from build123d import *

# Parameters (mm, degrees)
F0_R     = 41.275
F1_DEPTH = 1.524
F2_R     = 2.2479
F3_DEPTH = 1.524
F4_R     = 29.3751
F5_DEPTH = 1.524


with BuildPart() as f1:
    # F0 (on Top) → F1 (new body)
    with BuildSketch(Plane.XY):
        Circle(F0_R)
    extrude(amount=F1_DEPTH)

    # F2 (on face) → F3 (cut, through all)
    with BuildSketch(Plane.XY.offset(1.524)):
        with Locations((0, 36.5252)):
            Circle(F2_R)
        with Locations((-31.631751, 18.2626)):
            Circle(F2_R)
        with Locations((-31.631751, -18.2626)):
            Circle(F2_R)
        with Locations((0, -36.5252)):
            Circle(F2_R)
        with Locations((31.631751, -18.2626)):
            Circle(F2_R)
        with Locations((31.631751, 18.2626)):
            Circle(F2_R)
    extrude(amount=-F3_DEPTH, mode=Mode.SUBTRACT)

    # F4 (on face) → F5 (cut, through all)
    with BuildSketch(Plane.XY.offset(1.524)):
        Circle(F4_R)
    extrude(amount=-F5_DEPTH, mode=Mode.SUBTRACT)


solid = f1.part
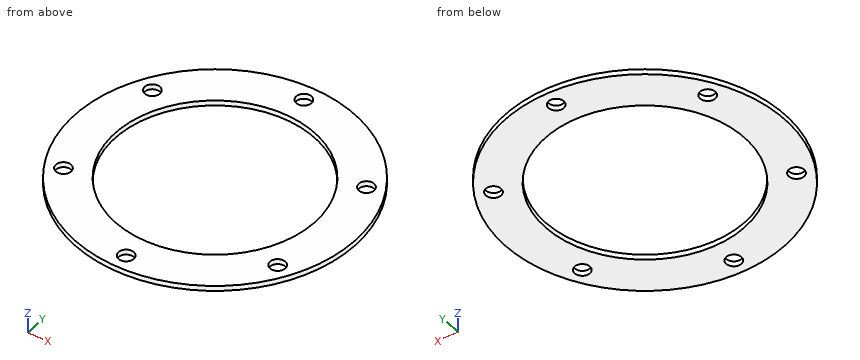
For this review, take the finished solid that the model builds, in its own axes (mm). Coordinates: 2 decimals unless noted, no trailing zeros. Loops run counter-clockwise (first coordinate to the right, second up) from the corner with the lowest first, then second, coordinate; pieces in that order, holes last. Notation, with made-up numbers: (1.5, 45.25) - (25.5, 45.25) arc R20 cw to (25.5, 55.25) - close; hole circle Ø7 at (84, 30). An arc over 180 degrees is marked (long way). Return JSON: item names as keys, results as strings.
Item 1: Take a section at C-C (z = 0.85). Give the boundary of the cut face in (x, y) (3 decimals), then the cut area to 3 significant figures.
Determined:
{"outline": "circle Ø82.55 at (0, 0); hole circle Ø4.496 at (-31.632, -18.263); hole circle Ø4.496 at (-31.632, 18.263); hole circle Ø58.75 at (0, 0); hole circle Ø4.496 at (0, -36.525); hole circle Ø4.496 at (0, 36.525); hole circle Ø4.496 at (31.632, -18.263); hole circle Ø4.496 at (31.632, 18.263)", "area": "2,550 mm2"}
Item 2: Take a section at A-A (y = 0). Give the boundary of the cut face in (x, z) (3 decimals), then the cut area to 3 significant figures.
Determined:
{"outline": "(-41.275, 0) - (-29.375, 0) - (-29.375, 1.524) - (-41.275, 1.524) - close; (29.375, 0) - (41.275, 0) - (41.275, 1.524) - (29.375, 1.524) - close", "area": "36.3 mm2"}
Item 3: Take a section at D-D (x = 32). Give the boundary of the cut face in (y, z).
Determined:
{"outline": "(-26.07, 0) - (-20.48, 0) - (-20.48, 1.52) - (-26.07, 1.52) - close; (-16.05, 0) - (16.05, 0) - (16.05, 1.52) - (-16.05, 1.52) - close; (20.48, 0) - (26.07, 0) - (26.07, 1.52) - (20.48, 1.52) - close"}
Item 4: Take a section at B-B (x = 0). Give the boundary of the cut face in (y, z) (3 decimals), then the cut area to 3 significant figures.
Determined:
{"outline": "(-41.275, 0) - (-38.773, 0) - (-38.773, 1.524) - (-41.275, 1.524) - close; (-34.277, 0) - (-29.375, 0) - (-29.375, 1.524) - (-34.277, 1.524) - close; (29.375, 0) - (34.277, 0) - (34.277, 1.524) - (29.375, 1.524) - close; (38.773, 0) - (41.275, 0) - (41.275, 1.524) - (38.773, 1.524) - close", "area": "22.6 mm2"}
Item 5: For line 1 (Y direction, x = 0, z = 1.05) (3 decimals); line 2 (X direction, y = -1, z = 0.9); line 3 (X direction, y = -16.5, z = 0.4), list the stretches that pass through material, from the lowest coordinate up.
Determined:
{"line 1": "y = -41.275 to -38.773, -34.277 to -29.375, 29.375 to 34.277, 38.773 to 41.275", "line 2": "x = -41.26 to -29.36, 29.36 to 41.26", "line 3": "x = -37.83 to -33.03, -30.24 to -24.3, 24.3 to 30.24, 33.03 to 37.83"}
